For this review, take the finished solid that the model builds, in its own axes (mm). A direction names the side the tool comes from. Round coordinates to 2 decimals unless told otherwise and drop trailing zeros. Order: outer loops, then holes, each group sorted by start corner. A loop starts at its lowest first (then second) coordinate and runs counter-clockwise, first axis right, second up. Notation, with made-up numbers: (-26.5, -19.75) -> (11.5, -19.75) arc R19 ccw to (11.5, 4.25) -> close; hole circle Ø4 at (56, 17.25). An arc over 180 degrees is marked (long way). Answer in a Markdown table with one row per item.
```python
from build123d import *

# Parameters (mm, degrees)
F0_R     = 7.4
F1_DEPTH = 45
F0_W     = 30
F0_H     = 30
F2_DEPTH = 30
F3_R     = 1


with BuildPart() as f1:
    # F0 (on Top) → F1 (new body)
    with BuildSketch(Plane.XY):
        with Locations((1.971214, -19.989052)):
            Circle(F0_R)
    extrude(amount=F1_DEPTH)

    # F0 (on Top) → F2 (join)
    with BuildSketch(Plane.XY):
        with Locations((1.971214, -19.989052)):
            Rectangle(F0_W, F0_H)
        with Locations((1.971214, -19.989052)):
            Circle(F0_R, mode=Mode.SUBTRACT)
    extrude(amount=F2_DEPTH)

    # F3
    f3_edges = [f1.edges().sort_by_distance(p)[0] for p in [
        (16.971214, -4.989052, 15),
        (-13.028786, -4.989052, 15),
        (1.971214, -4.989052, 0),
        (1.971214, -4.989052, 30),
        (-13.028786, -34.989052, 15),
        (-13.028786, -19.989052, 0),
        (-13.028786, -19.989052, 30),
        (16.971214, -34.989052, 15),
        (1.971214, -34.989052, 0),
        (1.971214, -34.989052, 30),
        (16.971214, -19.989052, 0),
        (16.971214, -19.989052, 30),
    ]]
    fillet(f3_edges, radius=F3_R)


solid = f1.part
```
Q1. Take a section at C-C, the plane x = 6.5. Write out the cut boundary in (y, z), then the cut area to 3 significant figures.
Answer key:
| item | result |
|---|---|
| outline | (-34.99, 1) arc R1 ccw to (-33.99, 0) -> (-5.99, 0) arc R1 ccw to (-4.99, 1) -> (-4.99, 29) arc R1 ccw to (-5.99, 30) -> (-14.14, 30) -> (-14.14, 45) -> (-25.84, 45) -> (-25.84, 30) -> (-33.99, 30) arc R1 ccw to (-34.99, 29) -> close |
| area | 1,070 mm^2 |
Q2. Take a section at D-D, the plane y = -23. Write out the cut boundary in (x, z).
Answer key:
| item | result |
|---|---|
| outline | (-13.03, 1) arc R1 ccw to (-12.03, 0) -> (15.97, 0) arc R1 ccw to (16.97, 1) -> (16.97, 29) arc R1 ccw to (15.97, 30) -> (8.73, 30) -> (8.73, 45) -> (-4.79, 45) -> (-4.79, 30) -> (-12.03, 30) arc R1 ccw to (-13.03, 29) -> close |
Q3. Take a section at B-B, the plane y = -32.25. Write out the cut boundary in (x, z), then the cut area to 3 significant figures.
Answer key:
| item | result |
|---|---|
| outline | (-13.03, 1) arc R1 ccw to (-12.03, 0) -> (15.97, 0) arc R1 ccw to (16.97, 1) -> (16.97, 29) arc R1 ccw to (15.97, 30) -> (-12.03, 30) arc R1 ccw to (-13.03, 29) -> close |
| area | 899 mm^2 |
Q4. Clearance check with flat-ended pins moving along their axes: pin 1 Ø4 at (y, z) = (-19.5, 38) entering from -X; pin 2 Ø3 at (x, y) = (8, -29) entering from +Z. State where each tip first meets the part, or that it passes through.
Answer key:
| item | result |
|---|---|
| pin 1 | stops at x = -5.43 |
| pin 2 | stops at z = 30 |
Q5. Tool access review of faces 1 (the face through (-12.74, -34.69, 15.2)), 2 (the face through (8, -14, 30)): name each direction out of +Z, -Z, +X, -X, +Y, -Y from which nothing blocks a thin tool from reaching the whole face with its end or side.
Answer key:
| item | result |
|---|---|
| face 1 | +Z, -Z, -X, -Y |
| face 2 | +Z |
Q6. To check wall thickness, follow probe 1 along Z at (x, y) = (-8.5, -32.5); probe 2 along X at (y, z) = (-20.5, 38.5). State the ranges of each line that lie inside material, in increasing order.
Answer key:
| item | result |
|---|---|
| probe 1 | z = 0 to 30 |
| probe 2 | x = -5.41 to 9.35 |
Q7. Take a section at A-A, the plane x = -7.25. Write out the cut boundary in (y, z), then the cut area to 3 significant figures.
Answer key:
| item | result |
|---|---|
| outline | (-34.99, 1) arc R1 ccw to (-33.99, 0) -> (-5.99, 0) arc R1 ccw to (-4.99, 1) -> (-4.99, 29) arc R1 ccw to (-5.99, 30) -> (-33.99, 30) arc R1 ccw to (-34.99, 29) -> close |
| area | 899 mm^2 |
